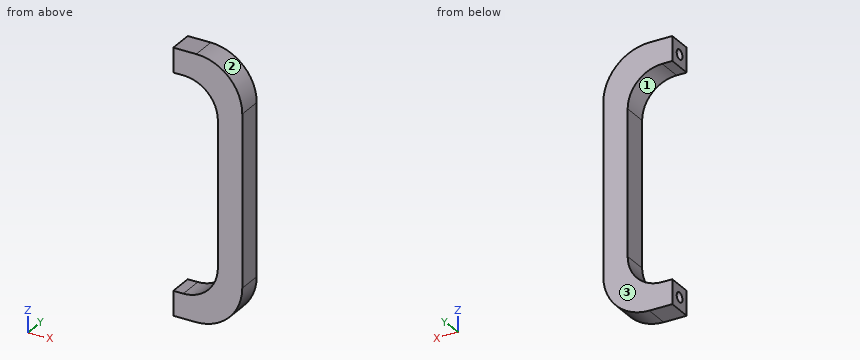
Autodesk Inventor part; units mm, degrees
ref_plane "YZ Plane" through (0, 0, 0) normal (1, 0, 0) x (0, 1, 0)
ref_plane "XZ Plane" through (0, 0, 0) normal (0, 1, 0) x (-1, 0, 0)
ref_plane "XY Plane" through (0, 0, 0) normal (0, 0, 1) x (1, 0, 0)
sketch "Sketch1" plane through (0, 0, 0) normal (0, 1, 0) x (-1, 0, 0)
  line L0 (15, 57) -> (-15, 57)
  line L1 (-15, 57) -> (-15, -57)
  line L2 (-15, -57) -> (15, -57)
  line L3 (15, -57) -> (15, 57)
  line L4 (0, 57) -> (0, -57) construction
  line L5 (15, 0) -> (-15, 0) construction
  line L6 (15, 46.3934) -> (10.6066, 46.3934)
  line L7 (-4.3934, 31.3934) -> (-4.3934, -31.3934)
  line L8 (10.6066, -46.3934) -> (15, -46.3934)
  line L9 (15, -46.3934) -> (15, 46.3934)
  arc A0 (10.6066, 46.3934) -> (-4.3934, 31.3934) centre (10.6066, 31.3934) ccw
  arc A1 (-4.3934, -31.3934) -> (10.6066, -46.3934) centre (10.6066, -31.3934) ccw
  point P0 (0, 0)
  point P1 (-4.3934, -46.3934)
  point P2 (-4.3934, 46.3934)
  dimension "d0" = 114
  dimension "d1" = 30
  dimension "d4" = 15
  dimension "d5" = 10.6066
  dimension "d17" = 92.7868
  dimension "d20" = 15
extrude "Extrusion1" add sketch "Sketch1" along normal blind 10.6066 contours L3 L6 A0 L7 A1 L8 L2 L1 L0
sketch "Sketch4" plane through (4.3934, 0, 46.3934) normal (-1, 0, 0) x (0, 0, 1)
  circle A0 centre (5.2379, 5.2459) radius 2.1
  circle A1 centre (-98.0247, 5.2459) radius 2.1
  line L0 (5.2379, 5.2459) -> (-98.0247, 5.2459)
  point P0 (-46.3934, 0)
  dimension "d18" = 103.2627
fillet "Fillet2" radius 20 2 edges at (15, 5.3033, 57) (15, 5.3033, -57)
hole "Hole2" at (4.3934, 5.2459, 51.6313) direction (-1, 0, 0) diameter 4.2 end through all
mirror "Mirror2" about plane through (0, 0, 0) normal (0, 0, 1) of "Hole2"
equation "\"d6\" = d5"
properties part number "acc door handle"
Verification items for the finished model (mm, model axes). Face numbers are marked on the shaded views. Give positions to 0.01 mm unless a question says otherwise; leave off trailing zeros. Write each loop counter-clockwise with the first axis right and the second up, starting at its lowest first coordinate (ties: lowest second). Pieces come first, ordered by that corner, then holes. Notation, with made-up numbers: (-20, 7.5) -> (-16, 7.5) arc R5 cw to (-16, 13.5) -> close; hole circle Ø6 at (-40, 21.25). An arc over 180 degrees is marked (long way). Use CSV: the item, a comma, the result in double quotes.
(1) Sectioned sample at D-D (z = 24). Record the cut outline in (x, y), plus the area to 4 significant figures.
Derived:
outline,"(4.39, 0) -> (15, 0) -> (15, 10.61) -> (4.39, 10.61) -> close"
area,"112.5 mm^2"
(2) Sectioned sample at A-A (y = 1.5). Record the cut outline in (x, z).
Derived:
outline,"(-15, -57) -> (-5, -57) arc R20 ccw to (15, -37) -> (15, 37) arc R20 ccw to (-5, 57) -> (-15, 57) -> (-15, 46.39) -> (-10.61, 46.39) arc R15 cw to (4.39, 31.39) -> (4.39, -31.39) arc R15 cw to (-10.61, -46.39) -> (-15, -46.39) -> close"
(3) Sectioned sample at B-B (x = -6). Record the cut outline in (y, z), plus the area to 3 significant figures.
Derived:
outline,"(0, -57) -> (10.61, -57) -> (10.61, -45.67) -> (0, -45.67) -> close; (0, 45.67) -> (10.61, 45.67) -> (10.61, 57) -> (0, 57) -> close; hole circle Ø4.2 at (5.25, -51.63); hole circle Ø4.2 at (5.25, 51.63)"
area,"213 mm^2"
(4) Material ranges on L1, parallel to Z at x = -10.5, y = 6.75; L2, parallel to Z at x = -2.5, y = 6; L3, parallel to X at y = 5, z = -2.5, recorded low to high.
Derived:
L1,"z = -57 to -53.1, -50.17 to -46.39, 46.39 to 50.17, 53.1 to 57"
L2,"z = -56.84 to -53.59, -49.67 to -44.01, 44.01 to 49.67, 53.59 to 56.84"
L3,"x = 4.39 to 15"
(5) Go/stop test with flat-tipped pins: pin 1 (8 mm diameter, centred on x = 0, z = 25, fed in from +Y); pin 2 (1 mm diameter, centred on y = 8, z = 40.5, fed in from -X); pin 3 (3 mm diameter, centred on x = 7, y = 1.5, fed in from +Z); pin 4 (6 mm diameter, centred on y = 6.5, z = 26.5, fed in from -X). Record where each tip stops, or that it passes through.
Derived:
pin 1,"passes through"
pin 2,"stops at x = 0.91"
pin 3,"stops at z = 54.02"
pin 4,"stops at x = 4.39"
(6) Sectioned sample at C-C (x = 11). Record the cut outline in (y, z).
Derived:
outline,"(0, -49) -> (10.61, -49) -> (10.61, 49) -> (0, 49) -> close"
(7) Release check for a two-part mould opening along Z. For the marked faces 1, 2 and 3 record: +Z half, -Z half, draft (parallel to the pull), parting line (faces both ways), or undercut.
Derived:
face 1,"undercut"
face 2,"+Z half"
face 3,"draft"
